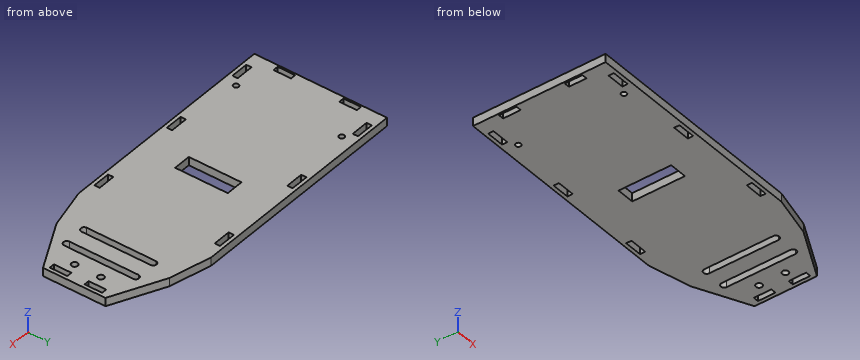
```python
from build123d import *

# Parameters (mm, degrees)
SKETCH1_W           = 181
SKETCH1_H           = 75.57
BOSS_EXTRUDE2_DEPTH = 4.75
SKETCH6_W           = 3
SKETCH6_H           = 10
SKETCH6_W_2         = 10.095812656
SKETCH6_H_2         = 3.003442242
SKETCH6_W_3         = 10
SKETCH6_H_3         = 30
SKETCH6_R           = 1.5
SKETCH6_R_2         = 1.85
SKETCH6_R_3         = 1.75
CUT_EXTRUDE7_DEPTH  = 9
CUT_EXTRUDE8_DEPTH  = 4.75


with BuildPart() as part:
    # Sketch1 → Boss-Extrude2 (new body)
    with BuildSketch(Plane.XY):
        Rectangle(SKETCH1_W, SKETCH1_H)
    extrude(amount=BOSS_EXTRUDE2_DEPTH)

    # Sketch6 → Cut-Extrude7 (cut)
    with BuildSketch(Plane.XY.offset(4.75)):
        Polygon((-81.955185068, 35.785), (-81.955183992, 32.802018857), (-71.81277502, 32.798644215), (-71.859372412, 35.785), align=None)
        with Locations((-88, 18.75)):
            Rectangle(SKETCH6_W, SKETCH6_H)
        with Locations((-88, -18.75)):
            Rectangle(SKETCH6_W, SKETCH6_H)
        Polygon((-34.13878131, 35.785), (-34.130786214, 32.798291399), (-24.042968654, 32.781557758), (-24.042968654, 35.785), align=None)
        Polygon((-71.81277502, -32.788413815), (-81.955183992, -32.785039173), (-81.955181828, -35.785039173), (-71.955181828, -35.785031959), align=None)
        Polygon((-33.95518398, -32.801010013), (-33.947153334, -35.800999264), (-23.947156396, -35.808824865), (-23.946905936, -32.804340026), align=None)
        with Locations((87, 9.9)):
            Rectangle(SKETCH6_W, SKETCH6_H)
        with Locations((24.004937674, 34.283278879)):
            Rectangle(SKETCH6_W_2, SKETCH6_H_2)
        Polygon((29.052844002, -32.806257253), (19.053094123, -32.805423656), (19.052844037, -35.805423646), (29.052844002, -35.806257264), align=None)
        with Locations((-8.31156853, 0)):
            Rectangle(SKETCH6_W_3, SKETCH6_H_3)
        with Locations((87, -9.9)):
            Rectangle(SKETCH6_W, SKETCH6_H)
        Polygon((61.466273892, -32.14), (38.055212144, -37.785), (90.5, -37.785), (90.5, -17.2), align=None)
        Polygon((61.46627389, 32.14), (90.5, 18.385572572), (90.5, 37.785), (38.055212144, 37.785), align=None)
        with Locations((-67.23, 30.095)):
            Circle(SKETCH6_R)
        with Locations((-67.23, -30.095)):
            Circle(SKETCH6_R)
        with Locations((70.00651733, -12.753407437)):
            Circle(SKETCH6_R_2)
        with Locations((70.00651733, 12.892480558)):
            Circle(SKETCH6_R_2)
        with Locations((70.00651733, 0)):
            Circle(SKETCH6_R_2)
        with Locations((57.30651733, 12.892480558)):
            Circle(SKETCH6_R_2)
        with Locations((57.30651733, 0)):
            Circle(SKETCH6_R_2)
        with Locations((57.30651733, -12.753407437)):
            Circle(SKETCH6_R_2)
        with Locations((79.833359723, -7.5)):
            Circle(SKETCH6_R_3)
        with Locations((79.833359723, 7.5)):
            Circle(SKETCH6_R_3)
    extrude(amount=-CUT_EXTRUDE7_DEPTH, mode=Mode.SUBTRACT)

    # Sketch9 → Cut-Extrude8 (cut)
    with BuildSketch(Plane.XY.offset(4.75)):
        with BuildLine():
            Line((59.15651733, 19.742480558), (59.15651733, -19.603407437))
            ThreePointArc((59.15651733, -19.603407437), (57.30651733, -21.453407437), (55.45651733, -19.603407437))
            Line((55.45651733, -19.603407437), (55.45651733, 19.742480558))
            ThreePointArc((55.45651733, 19.742480558), (57.30651733, 21.592480558), (59.15651733, 19.742480558))
        make_face()
        with BuildLine():
            Line((71.85651733, 19.742480558), (71.85651733, -19.603407437))
            ThreePointArc((71.85651733, -19.603407437), (70.00651733, -21.453407437), (68.15651733, -19.603407437))
            Line((68.15651733, -19.603407437), (68.15651733, 19.742480558))
            ThreePointArc((68.15651733, 19.742480558), (70.00651733, 21.592480558), (71.85651733, 19.742480558))
        make_face()
    extrude(amount=-CUT_EXTRUDE8_DEPTH, mode=Mode.SUBTRACT)


solid = part.part
```
The model under review builds one solid part; all positions refer to its coordinate system, in mm. Coordinates: 2 decimals unless noted, no trailing zeros. Write each loop counter-clockwise with the first axis right and the second up, starting at its lowest first coordinate (ties: lowest second). Pieces come first, ordered by that corner, then holes. Notation, with made-up numbers: (76, 68) -> (96, 68) arc R30 ccw to (96, 103) -> close; hole circle Ø3 at (77, 40.5). An arc over 180 degrees is marked (long way). One line per item, written item: value. Start each with the question number.
Q1. Clearance check with a flat-ended pin moving along its axis: P1, Ø1.4, axis at y = 20, z = 2.5, coming from the +X side. State where the tip first meets the part, or that it passes through.
Q2. Add section B-B, the plane z = 1.7. Count the separate pieces of the cut face and the enclosed holes in it, then the cut area to 3 significant figures.
Q3. To check wall thickness, follow probe 1 along Y at (x, z) = (-67.23, 2) (3 decimals); probe 2 along Y at (x, z) = (24.5, 2.85) (3 decimals); probe 3 along X at (y, z) = (15.5, 2.7). State the ranges of each line that lie inside material, in increasing order.
Q4. Add section A-A, the plane y = -7.5. Give the boundary of the cut face in (x, z).
Q5. Add section C-C, the plane x = 46. Give the boundary of the cut face in (y, z), then the cut area to 3 significant figures.
Response:
1. P1: x = 88.57
2. separate pieces: 1
2. enclosed holes: 17
2. area: 11,900 mm²
3. probe 1: -37.785 to -31.595, -28.595 to 28.595, 31.595 to 37.785
3. probe 2: -37.785 to -35.806, -32.806 to 32.782, 35.785 to 37.785
3. probe 3: -90.5 to -89.5, -86.5 to 55.46, 59.16 to 68.16, 71.86 to 90.5
4. outline: (-90.5, 0) -> (-13.31, 0) -> (-13.31, 4.75) -> (-90.5, 4.75) -> close; (-3.31, 0) -> (55.46, 0) -> (55.46, 4.75) -> (-3.31, 4.75) -> close; (59.16, 0) -> (68.16, 0) -> (68.16, 4.75) -> (59.16, 4.75) -> close; (71.86, 0) -> (78.08, 0) -> (78.08, 4.75) -> (71.86, 4.75) -> close; (81.58, 0) -> (85.5, 0) -> (85.5, 4.75) -> (81.58, 4.75) -> close; (88.5, 0) -> (90.5, 0) -> (90.5, 4.75) -> (88.5, 4.75) -> close
5. outline: (-35.87, 0) -> (35.87, 0) -> (35.87, 4.75) -> (-35.87, 4.75) -> close
5. area: 341 mm²
